Design review of the part shown in the three views and the two pictorial views. Dimensions are in mm from the part's minimum x, y and z. Round coordinates to 2 decimals unless told otherwise and drop trailing zeros. Write each loop counter-clockwise with the first axis right and the second up, starting at its lowest first coordinate (ties: lowest second). Pieces come first, ordered by that corner, then holes. Notation, with made-up numbers: (89, 86.25) - (109, 86.25) arc R20 cw to (109, 105.25) - close; hole circle Ø5 at (44, -8). An arc over 180 degrees is marked (long way). Use one line per item in the form item = value.
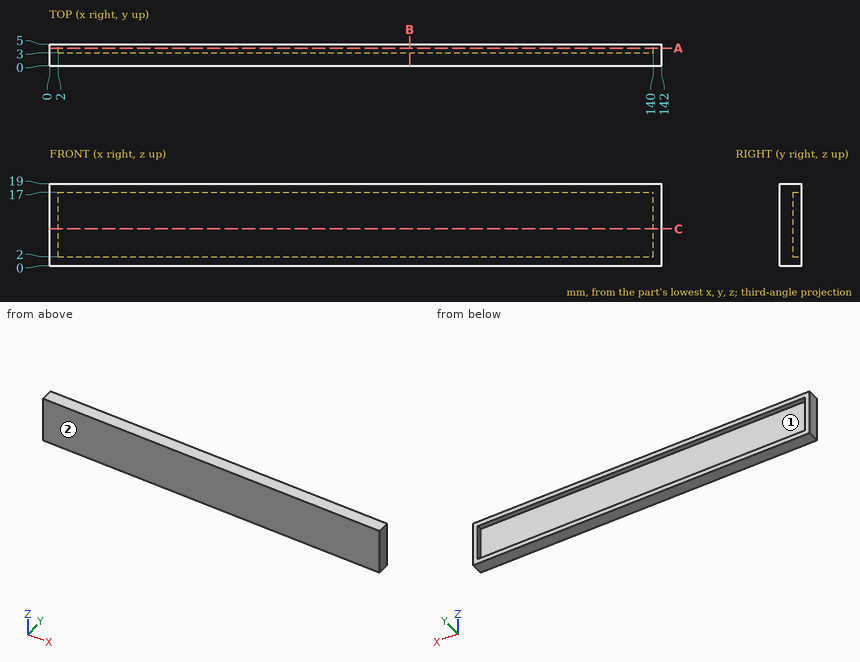
(1) To check wall thickness, follow L1, parallel to X at y = 3.95, z = 13.5; L2, parallel to Z at x = 114.5, y = 4.1; L3, parallel to Y at x = 61, z = 6.5. State the ranges of each line that lie inside material, in increasing order.
Geometry results:
L1 = 0 to 2, 140 to 142
L2 = 0 to 2, 17 to 19
L3 = 0 to 3
(2) The part is to be moulded in two halves that separate along X. For the marked faces 1 and 2, say which applies: +X half, -X half, draft (parallel to the pull), parting line (faces both ways), or undercut.
Geometry results:
face_1 = undercut
face_2 = draft
(3) Insertion check: P1, Ø3, axis at x = 79, z = 11, coming from the +Y side; P2, Ø2, axis at y = 4, z = 11.5, coming from the -X side. Each pin has a flat end and moves straight along its axis. Give the tip position at first contact, or say it passes through.
Geometry results:
P1 = 3
P2 = 0
(4) Add section B-B on x = 83.5. Write out the cut boundary in (y, z), then the cut area to 3 significant figures.
Geometry results:
outline = (0, 0) - (5, 0) - (5, 2) - (3, 2) - (3, 17) - (5, 17) - (5, 19) - (0, 19) - close
area = 65.0 mm2
(5) Add section A-A on y = 4.05. Write out the cut boundary in (x, z), then the cut area to 3 significant figures.
Geometry results:
outline = (0, 0) - (142, 0) - (142, 19) - (0, 19) - close; hole (2, 2) - (140, 2) - (140, 17) - (2, 17) - close
area = 628 mm2
(6) Add section C-C on z = 8.5. Write out the cut boundary in (x, y).
Geometry results:
outline = (0, 0) - (142, 0) - (142, 5) - (140, 5) - (140, 3) - (2, 3) - (2, 5) - (0, 5) - close
